Here's how the part is built. I have some questions about the finished solid (model axes, mm). A direction names the side the tool comes from. Coordinates: 2 decimals unless noted, no trailing zeros. Write each loop counter-clockwise with the first axis right and the second up, starting at its lowest first coordinate (ties: lowest second). Pieces come first, ordered by that corner, then holes.
Item 1: I want a section at A-A (y = -19). Please give me the cut outline in (x, z), and give its area (3 significant figures).
Item 2: I'm going to push flat-ended pins straight in: P1, Ø4, axis at x = -15, z = 55, coming from the +Y side; P2, Ø8, axis at x = -5, y = 22.5, coming from the +Z side; P3, Ø15, axis at x = -2.5, z = 42, coming from the -Y side. Where does each tip first touch, or does it pass through?
Item 3: I want a section at C-C (x = 5). Please give me the cut outline in (y, z), and give its area (3 significant figures).
Item 4: I want a section at B-B (z = 6). Please give me the cut outline in (x, y), and give its area (3 significant figures).
Item 5: If we mould it in two halves opening along X, with no side actions, what happens to faces 1 (the face through (28, -17, 50)), 2 (the face through (3, -7.309, 35)), 3 (the face through (20.868, 5.086, 52.745))? For each: pulls with the +X half, pulls with the -X half, needs draft (parallel to the pull), parting line crosses it, or undercut.
Item 6: I want a section at D-D (y = 23). Please give me the cut outline in (x, z).
Item 7: Please list where these lines run through material, in increasing order: line 1 (X direction, y = -15, z = 57); line 2 (Z direction, x = 26.5, y = -19); line 3 (Z direction, x = -21, y = 5).
Item 8: For faces 4 (the face through (28, -12.309, 35)), 5 (the face through (18.123, -12, 35)), 6 (the face through (-14.132, 5.296, 52.745)), which set-ups out of +Z, -Z, +X, -X, +Y, -Y let a thin tool reach every point of the face, with its end or its side?
from build123d import *

# Parameters (mm, degrees)
IZIM1_W                     = 70
IZIM1_H                     = 50
Y_KSEKLIK_EKSTR_ZYON2_DEPTH = 70
IZIM2_W                     = 30
IZIM2_H                     = 10
KES_EKSTR_ZYON1_DEPTH       = 70
IZIM7_W                     = 30
IZIM7_H                     = 15
KES_EKSTR_ZYON3_DEPTH       = 70
KES_EKSTR_ZYON4_DEPTH       = 35
IZIM9_W                     = 15
IZIM9_H                     = 10
KES_EKSTR_ZYON5_DEPTH       = 70


with BuildPart() as part:
    # Çizim1 → Yükseklik-Ekstrüzyon2 (new body)
    with BuildSketch(Plane.XY):
        with Locations((3.122705421, 2.690839695)):
            Rectangle(IZIM1_W, IZIM1_H)
    extrude(amount=Y_KSEKLIK_EKSTR_ZYON2_DEPTH)

    # Çizim2 → Kes-Ekstrüzyon1 (cut)
    with BuildSketch(Plane.ZY.offset(31.877294579)):
        with Locations((35, -17.309160305)):
            Rectangle(IZIM2_W, IZIM2_H)
    extrude(amount=-KES_EKSTR_ZYON1_DEPTH, mode=Mode.SUBTRACT)

    # Çizim7 → Kes-Ekstrüzyon3 (cut)
    with BuildSketch(Plane.XY.offset(70)):
        with Locations((3.122705421, -14.809160305)):
            Rectangle(IZIM7_W, IZIM7_H)
    extrude(amount=-KES_EKSTR_ZYON3_DEPTH, mode=Mode.SUBTRACT)

    # Çizim8 → Kes-Ekstrüzyon4 (cut)
    with BuildSketch(Plane.XY.offset(70)):
        Polygon((38.122705421, -2.309160305), (3.122705421, 12.690839695), (-31.877294579, -2.309160305), (-31.877294579, 27.690839695), (38.122705421, 27.690839695), align=None)
    extrude(amount=-KES_EKSTR_ZYON4_DEPTH, mode=Mode.SUBTRACT)

    # Çizim9 → Kes-Ekstrüzyon5 (cut)
    with BuildSketch(Plane.ZY.offset(31.877294579)):
        with Locations((27.5, 22.690839695)):
            Rectangle(IZIM9_W, IZIM9_H)
    extrude(amount=-KES_EKSTR_ZYON5_DEPTH, mode=Mode.SUBTRACT)


solid = part.part
Answer:
1. outline: (-31.88, 0) - (-11.88, 0) - (-11.88, 20) - (-31.88, 20) - close; (-31.88, 50) - (-11.88, 50) - (-11.88, 70) - (-31.88, 70) - close; (18.12, 0) - (38.12, 0) - (38.12, 20) - (18.12, 20) - close; (18.12, 50) - (38.12, 50) - (38.12, 70) - (18.12, 70) - close
1. area: 1,600 mm2
2. P1: stops at y = 5.78
2. P2: stops at z = 20
2. P3: stops at y = -7.31
3. outline: (-7.31, 0) - (27.69, 0) - (27.69, 20) - (17.69, 20) - (17.69, 35) - (11.89, 35) - (11.89, 70) - (-7.31, 70) - close
3. area: 1,750 mm2
4. outline: (-31.88, -22.31) - (-11.88, -22.31) - (-11.88, -7.31) - (18.12, -7.31) - (18.12, -22.31) - (38.12, -22.31) - (38.12, 27.69) - (-31.88, 27.69) - close
4. area: 3,050 mm2
5. face 1: needs draft
5. face 2: undercut
5. face 3: pulls with the +X half
6. outline: (-31.88, 0) - (38.12, 0) - (38.12, 20) - (-31.88, 20) - close
7. line 1: x = -31.88 to -11.88, 18.12 to 38.12
7. line 2: z = 0 to 20, 50 to 70
7. line 3: z = 0 to 35
8. face 4: +X, -X, -Y
8. face 5: +Z, -Z, -Y
8. face 6: +Z, -X, +Y
